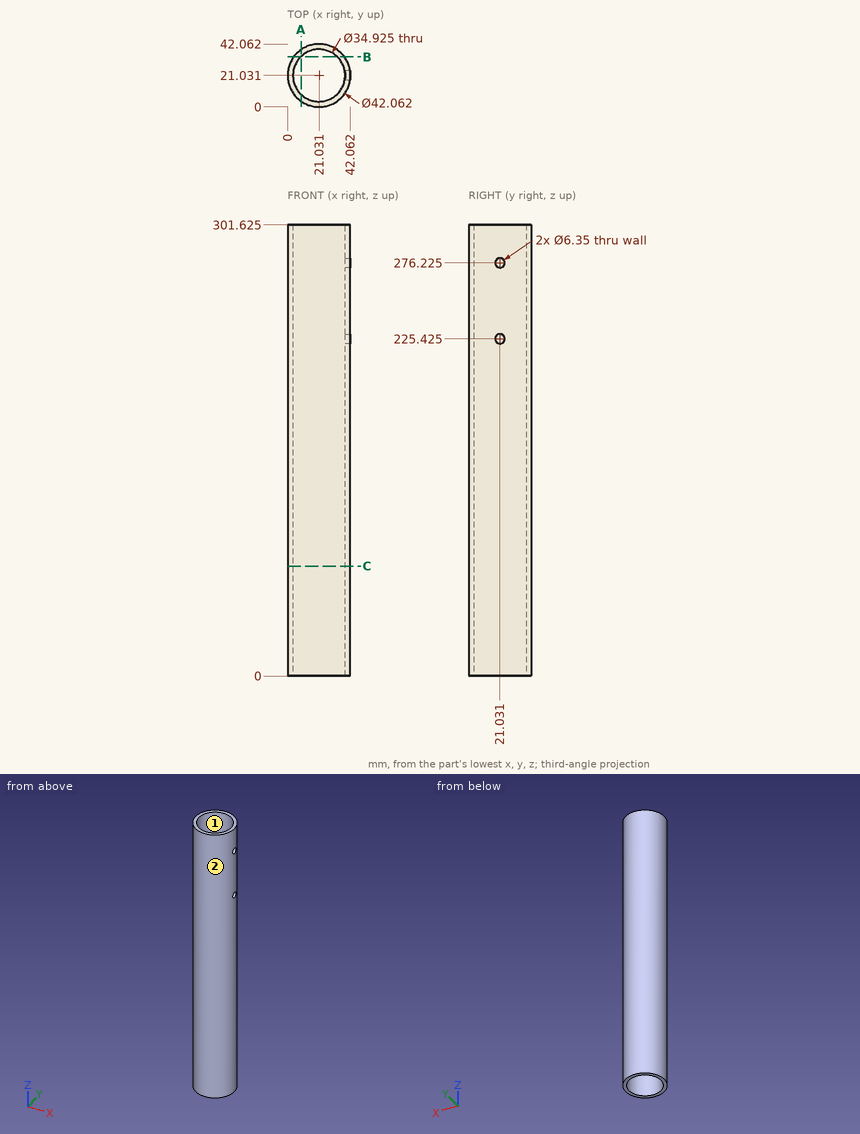
Answer from the drawing. Dimensions are ordinates in mm from the lowest x, y and z of the part. Coordinates: 2 decimals unless noted, no trailing zeros. Write each loop counter-clockwise with the first axis right and the second up, starting at its lowest first coordinate (ties: lowest second). Pieces come first, ordered by that corner, then holes. Notation, with made-up numbers: (-36.5, 46) - (-7.5, 46) arc R26 cw to (-7.5, 61) - close; hole circle Ø2 at (38, 32.5). An arc over 180 degrees is marked (long way). Answer as CSV lines item,"result".
1. Given P1, Ø6, axis at y = 7, z = 187.5, coming from the -X side (1 decimal); P2, Ø3, axis at y = 11, z = 63, coming from the -X side; P3, Ø1.5, axis at y = 32.5, z = 261, coming from the +X side (1 decimal), each flat-ended and moving along its own axis, determine where each tip first touches the part or whether it passes through.
Computed values:
P1,"stops at x = 3.1"
P2,"stops at x = 1.81"
P3,"stops at x = 39.1"
2. Find section A-A (x = 9). Give the vertices of the cut face in (y, z) (1 decimal).
Computed values:
outline,"(3.8, 0) - (8.4, 0) - (8.4, 301.6) - (3.8, 301.6) - close; (33.7, 0) - (38.3, 0) - (38.3, 301.6) - (33.7, 301.6) - close"
3. Find section C-C (z = 73.5). Give the vertices of the cut face in (x, y) (1 decimal).
Computed values:
outline,"circle Ø42.1 at (21, 21); hole circle Ø34.9 at (21, 21)"
4. Find section B-B (y = 33.5). Give the vertices of the cut face in (x, z) (1 decimal).
Computed values:
outline,"(4.1, 0) - (8.8, 0) - (8.8, 301.6) - (4.1, 301.6) - close; (33.3, 0) - (38, 0) - (38, 301.6) - (33.3, 301.6) - close"
5. Determine the mould class of the marked faces 1 and 2 for opening direction Y: +Y half, -Y half, draft (parallel to the pull), parting line (faces both ways), or undercut.
Computed values:
face 1,"undercut"
face 2,"parting line"
6. Straight lines are drawn through the part: line 1 (Z direction, x = 40, y = 22.5) (1 decimal); line 2 (Y direction, x = 20, z = 246) (1 decimal); line 3 (X direction, y = 7.5, z = 36) (1 decimal). For each, find the intervals that lie inside material, in ascending order. Write a range as [from, to].
Computed values:
line 1,"z = [0, 222.6], [228.2, 273.4], [279, 301.6]"
line 2,"y = [0, 3.6], [38.5, 42]"
line 3,"x = [4.9, 10], [32.1, 37.1]"
